Can you work these out from the model? Positions are in its coordinate system, mm. A direction names the side the tool comes from. Round coordinates to 2 decimals unless told otherwise and drop trailing zeros. Order: outer loops, then holes, each group sorted by start corner. A loop starts at its lowest first (then second) coordinate and runs counter-clockwise, first axis right, second up. Notation, with made-up numbers: M 89,-16 L 138,-16 A15 ccw 138,8 Z; hole C 76.25,42 d9. An arc over 180 degrees is marked long. Answer as a JSON object with one key per item and string values. Group by question number.
from build123d import *

# Parameters (mm, degrees)
SKETCH1_W                        = 12.7
SKETCH1_H                        = 25.4
SKETCH1_W_2                      = 101.6
SKETCH1_H_2                      = 63.5
BOSS_EXTRUDE1_DEPTH              = 12.7
F_1_4_20_TAPPED_HOLE1_AT_2_COUNT = 2
F_1_4_20_TAPPED_HOLE1_AT_2_PITCH = 38.1
CUT_EXTRUDE1_DEPTH               = 13.7
FILLET1_R                        = 3.175
FILLET2_R                        = 3.175


with BuildPart() as part:
    # Sketch1 → Boss-Extrude1 (new body)
    with BuildSketch(Plane.XY):
        with Locations((-57.15, 0)):
            Rectangle(SKETCH1_W, SKETCH1_H)
        Rectangle(SKETCH1_W_2, SKETCH1_H_2)
        with Locations((57.15, 0)):
            Rectangle(SKETCH1_W, SKETCH1_H)
    extrude(amount=BOSS_EXTRUDE1_DEPTH)

    # Sketch2 → 1/4-20 Tapped Hole1 (revolve, cut)
    with BuildSketch(Plane(origin=(50.8, 19.05, 6.35), x_dir=(0, 0, -1), z_dir=(0, 1, 0))):
        Polygon((0, 0), (0, 18.043816902), (2.5527, 16.51), (2.5527, 12.7), (3.175, 12.7), (3.175, 0), align=None)
    f_1_4_20_tapped_hole1 = revolve(axis=Axis((57.15, 19.05, 6.35), (-1, 0, 0)), mode=Mode.SUBTRACT)

    # 1/4-20 Tapped Hole1 at 2: 1/4-20 Tapped Hole1 ×2
    with Locations(*[(0, -i * F_1_4_20_TAPPED_HOLE1_AT_2_PITCH, 0) for i in range(1, F_1_4_20_TAPPED_HOLE1_AT_2_COUNT)]):
        add(f_1_4_20_tapped_hole1, mode=Mode.SUBTRACT)

    # Mirror1: 1/4-20 Tapped Hole1 across plane
    add(f_1_4_20_tapped_hole1.mirror(Plane(origin=(0, 0, 0), x_dir=(0, 0, 1), z_dir=(1, 0, 0))), mode=Mode.SUBTRACT)

    # Mirror1 copy 1 sketch → Mirror1 copy 1 (revolve, cut)
    with BuildSketch(Plane(origin=(-50.8, -19.05, 6.35), x_dir=(0, 0, -1), z_dir=(0, 1, 0))):
        Polygon((0, 0), (0, -18.043816902), (2.5527, -16.51), (2.5527, -12.7), (3.175, -12.7), (3.175, 0), align=None)
    revolve(axis=Axis((-57.15, -19.05, 6.35), (-1, 0, 0)), mode=Mode.SUBTRACT)

    # Sketch4 → Cut-Extrude1 (cut, through all)
    with BuildSketch(Plane.XY.offset(12.7)):
        Polygon((-44.45, 0), (0, 19.05), (44.45, 0), (0, -19.05), align=None)
    extrude(amount=-CUT_EXTRUDE1_DEPTH, mode=Mode.SUBTRACT)

    # Fillet1
    fillet1_edges = [part.edges().sort_by_distance(p)[0] for p in [
        (0, 19.05, 6.35),
        (44.45, 0, 6.35),
        (0, -19.05, 6.35),
        (-44.45, 0, 6.35),
    ]]
    fillet(fillet1_edges, radius=FILLET1_R)

    # Fillet2
    fillet2_edges = [part.edges().sort_by_distance(p)[0] for p in [
        (-50.8, 31.75, 6.35),
        (50.8, 31.75, 6.35),
        (50.8, -31.75, 6.35),
        (-50.8, -31.75, 6.35),
    ]]
    fillet(fillet2_edges, radius=FILLET2_R)


solid = part.part
Item 1: I need wall thicknesses on line 1 (Y direction, x = 41.25, z = 6.35) (3 decimals); line 2 (Z direction, x = 41.75, y = 19.05) (3 decimals); line 3 (Y direction, x = 35.3, z = 6.35). Which ranges of each line are inside material? Lowest first, please.
Item 2: Suppose I cut it at B-B, the plane x = -16. Write out the boundary of the cut face in (y, z).
Item 3: I'm going to push flat-ended pins straight in: pin 1 Ø4.5 at (y, z) = (19.05, 6.35) entering from +X; pin 2 Ø6.5 at (x, z) = (-54.5, 8) entering from +Y; pin 3 Ø7 at (y, z) = (-19.5, 7.5) entering from +X. Where does each tip first touch, or does it pass through?
Item 4: On a 3-axis mill with a long thin cutter (end or side, diameter ignored), from which of +Z, -Z, +X, -X, +Y, -Y can I reach the whole of each face in a straight line? I mean faces 4 (the face through (57, 12.7, 6)), 5 (the face through (36.222, -16.558, 6.903)), 6 (the face through (19.191, 10.825, 6.439)). Say none if no direction works.
Item 5: If we mould it in two halves opening along X, with no side actions, what happens to faces 1 (the face through (-36.222, 16.898, 4.978)), 2 (the face through (-0.02, -18.77, 6.26)), 3 (the face through (63.5, 0, 6))? For each: +X half, -X half, draft (parallel to the pull), parting line (faces both ways), or undercut.
Item 6: Suppose I cut it at C-C, the plane y = 27. Write out the boundary of the cut face in (x, z), and give its area (3 significant figures).
Item 7: Suppose I cut it at A-A, the plane y = 0. Write out the boundary of the cut face in (x, z).
Computed:
{
 "1": {"line 1": "y = -31.75 to -22.225, -15.875 to 15.875, 22.225 to 31.75", "line 2": "z = 0 to 3.175, 9.525 to 12.7", "line 3": "y = -31.75 to -21.6, -16.5 to -3.92, 3.92 to 16.5, 21.6 to 31.75"},
 "2": {"outline": "M -31.75,0 L -12.19,0 L -12.19,12.7 L -31.75,12.7 Z; M 12.19,0 L 31.75,0 L 31.75,12.7 L 12.19,12.7 Z"},
 "3": {"pin 1": "stops at x = 34.11", "pin 2": "stops at y = 12.7", "pin 3": "stops at x = 50.8"},
 "4": {"face 4": "+Z, -Z, +X, +Y", "face 5": "+X", "face 6": "+Z, -Z"},
 "5": {"face 1": "draft", "face 2": "undercut", "face 3": "+X half"},
 "6": {"outline": "M -50.8,0 L 50.8,0 L 50.8,12.7 L -50.8,12.7 Z", "area": "1,290 mm^2"},
 "7": {"outline": "M -63.5,0 L -39.56,0 L -39.56,12.7 L -63.5,12.7 Z; M 39.56,0 L 63.5,0 L 63.5,12.7 L 39.56,12.7 Z"}
}
